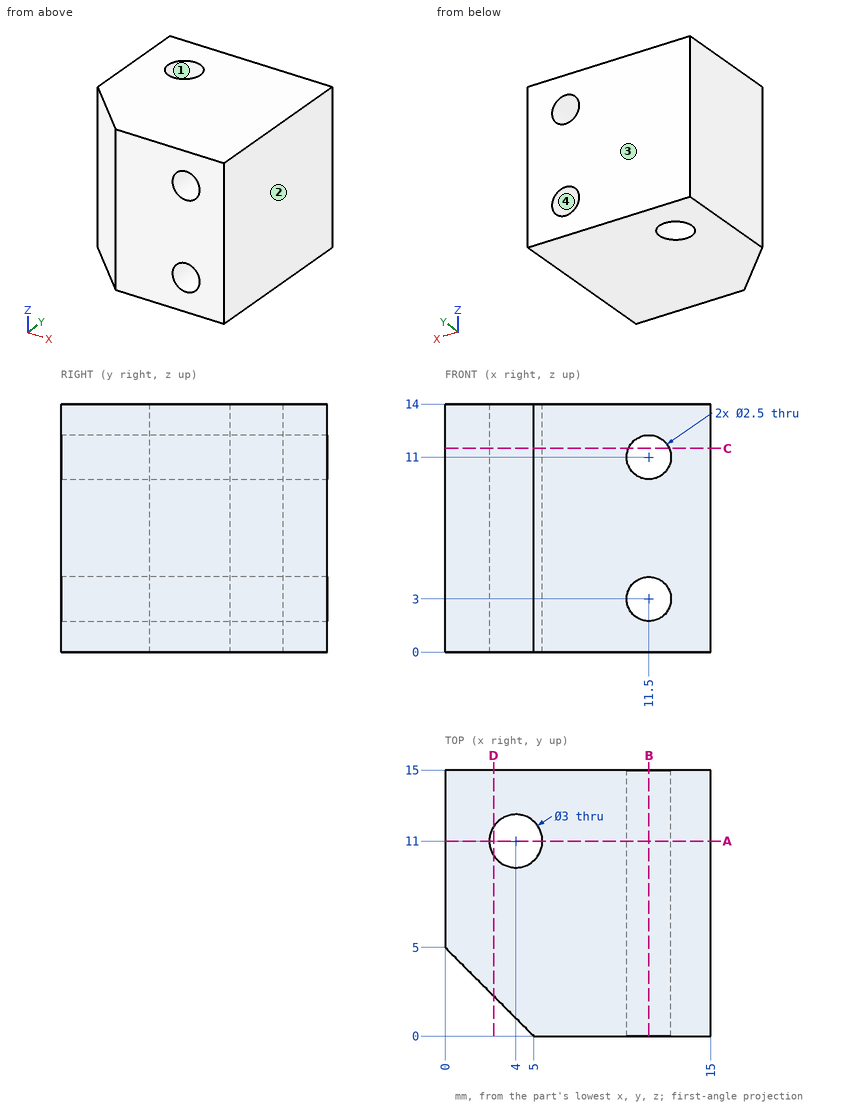
Job drawing, mm, ordinate dimensions from the low corner. One solid piece. Coordinates: 2 decimals unless noted, no trailing zeros. Order: outer loops, then holes, each group sorted by start corner. A loop starts at its lowest first (then second) coordinate and runs counter-clockwise, first axis right, second up. Notation, with made-up numbers: M -20.75,9 L 30.25,9 A18 ccw 30.25,36 Z; hole C 63.5,36 d1. An arc over 180 degrees is marked long. One line per question, with ' | ' between items.
Q1. Slice it at A-A (y = 11). Give the cut face in (x, z).
A:
outline: M 0,0 L 2.5,0 L 2.5,14 L 0,14 Z; M 5.5,0 L 15,0 L 15,14 L 5.5,14 Z; hole C 11.5,3 d2.5; hole C 11.5,11 d2.5
Q2. Slice it at D-D (x = 2.75). Give the cut face in (y, z).
A:
outline: M 2.25,0 L 10.17,0 L 10.17,14 L 2.25,14 Z; M 11.83,0 L 15,0 L 15,14 L 11.83,14 Z
Q3. Slice it at C-C (z = 11.5). Give the cut face in (x, y), and give its area (3 significant figures).
A:
outline: M 0,5 L 5,0 L 10.35,0 L 10.35,15 L 0,15 Z; M 12.65,0 L 15,0 L 15,15 L 12.65,15 Z; hole C 4,11 d3 | area: 171 mm^2
Q4. Two-plate mould, pull along X, no slides. Class the marked faces 1, 2, 3 and 4: +X half, -X half, draft (parallel to the pull), parting line (faces both ways), or undercut.
A:
face 1: undercut | face 2: +X half | face 3: draft | face 4: undercut
Q5. Slice it at B-B (x = 11.5). Give the cut face in (y, z), and give its area (3 significant figures).
A:
outline: M 0,0 L 15,0 L 15,1.75 L 0,1.75 Z; M 0,4.25 L 15,4.25 L 15,9.75 L 0,9.75 Z; M 0,12.25 L 15,12.25 L 15,14 L 0,14 Z | area: 135 mm^2
Q6. Drill centre lines: line 1 (Z direction, x = 12.5, y = 8.5); line 2 (X direction, y = 12.75, z = 11); line 3 (Z direction, x = 11.25, y = 6.5). Where is each one in solid material? Low to high.
A:
line 1: z = 0 to 2.25, 3.75 to 10.25, 11.75 to 14 | line 2: x = 0 to 10.25, 12.75 to 15 | line 3: z = 0 to 1.78, 4.22 to 9.78, 12.22 to 14
